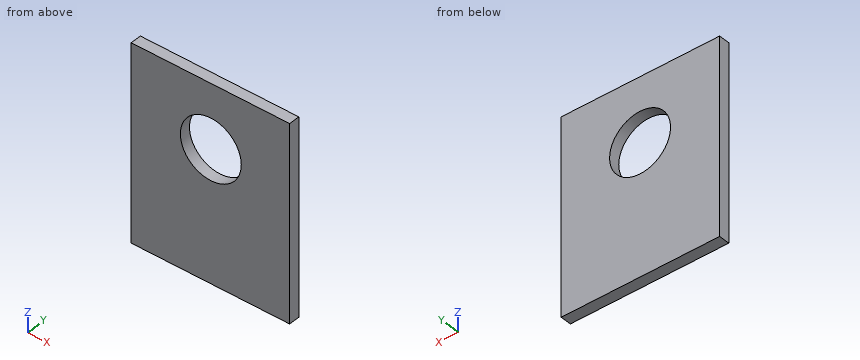
```python
from build123d import *

# Parameters (mm, degrees)
SKETCH011_R  = 50
PAD009_DEPTH = 40
BOX003_W     = 260
BOX003_H     = 18
BOX003_DEPTH = 320


with BuildPart() as body009:
    # Sketch011 → Pad009 (new body)
    with BuildSketch(Plane.XZ):
        with Locations((98.600952, 204.673477)):
            Circle(SKETCH011_R)
    extrude(amount=PAD009_DEPTH)


with BuildPart() as body009_1:
    # Body009 placement: moved
    add(body009.part.moved(Location((0, -212, 0))))


with BuildPart() as obj1:
    # Box003 → Box003 (new body)
    with BuildSketch(Plane(origin=(-32, -247, -10), x_dir=(1, 0, 0), z_dir=(0, 0, 1))):
        with Locations((130, 9)):
            Rectangle(BOX003_W, BOX003_H)
    extrude(amount=BOX003_DEPTH)

    # Cut003: cut Body009
    add(body009_1.part, mode=Mode.SUBTRACT)


solid = obj1.part
```
For this review, take the finished solid that the model builds, in its own axes (mm). Round coordinates to 2 decimals unless told otherwise and drop trailing zeros. Write each loop counter-clockwise with the first axis right and the second up, starting at its lowest first coordinate (ties: lowest second). Pieces come first, ordered by that corner, then holes. Notation, with made-up numbers: (78, 28.25) - (84, 28.25) arc R21 ccw to (84, 34.25) - close; hole circle Ø1 at (-35.5, 6.5). An arc over 180 degrees is marked (long way). Put each result on its own line as item: value.
Q1. We need section A-A (z = 196). Give the boundary of the cut face in (x, y).
Solved:
outline: (-32, -247) - (49.36, -247) - (49.36, -229) - (-32, -229) - close; (147.84, -247) - (228, -247) - (228, -229) - (147.84, -229) - close
Q2. We need section B-B (x = 106.5). Give the boundary of the cut face in (y, z).
Solved:
outline: (-247, -10) - (-229, -10) - (-229, 155.3) - (-247, 155.3) - close; (-247, 254.05) - (-229, 254.05) - (-229, 310) - (-247, 310) - close
Q3. We need section C-C (y = -241.5). Give the boundary of the cut face in (x, z).
Solved:
outline: (-32, -10) - (228, -10) - (228, 310) - (-32, 310) - close; hole circle Ø100 at (98.6, 204.67)
Q4. Wall thickness on probe 1 along Z at (x, y) = (99, -232.25); probe 2 along Z at (x, y) = (57.5, -229.75); probe 3 along X at (y, z) = (-230.5, 212): over which ranges is each line inside the solid? List them lowest first.
Solved:
probe 1: z = -10 to 154.68, 254.67 to 310
probe 2: z = -10 to 176.2, 233.15 to 310
probe 3: x = -32 to 49.14, 148.06 to 228
